Verification items for the finished model (mm, model axes). A direction names the side the tool comes from. Give positions to 0.01 mm unless a question says otherwise; leave off trailing zeros. Loops run counter-clockwise (first coordinate to the right, second up) from the corner with the lowest first, then second, coordinate; pieces in that order, holes last. Notation, with made-up numbers: M 24.5,-38.75 L 56.5,-38.75 A31 ccw 56.5,-9.75 Z; hole C 78,-37.5 d3. An arc over 180 degrees is marked long. Put each result on its own line as item: value. Start each with the question number.
from build123d import *

# Parameters (mm, degrees)
SKETCH1_R             = 60
BOSS_EXTRUDE1_DEPTH   = 19
SKETCH2_R             = 55
SKETCH2_R_2           = 50
CUT_EXTRUDE1_DEPTH    = 5
SKETCH6_W             = 17.5
SKETCH6_H             = 14
M6_TAPPED_HOLE1_D     = 5
M6_TAPPED_HOLE1_DEPTH = 15
M6_TAPPED_HOLE1_TIP   = 1.502151548


with BuildPart() as part:
    # Sketch1 → Boss-Extrude1 (new body)
    with BuildSketch(Plane(origin=(0, 0, 0), x_dir=(1, 0, 0), z_dir=(0, 1, 0))):
        with Locations(Location((0, 0, 0), (0, 0, 270))):
            Circle(SKETCH1_R)
    extrude(amount=BOSS_EXTRUDE1_DEPTH)

    # Sketch2 → Cut-Extrude1 (cut)
    with BuildSketch(Plane(origin=(0, 19, 0), x_dir=(1, 0, 0), z_dir=(0, 1, 0))):
        with Locations(Location((0, 0, 0), (0, 0, 270))):
            Circle(SKETCH2_R)
        with Locations(Location((0, 0, 0), (0, 0, 270))):
            Circle(SKETCH2_R_2, mode=Mode.SUBTRACT)
    extrude(amount=-CUT_EXTRUDE1_DEPTH, mode=Mode.SUBTRACT)

    # Sketch4 → Cut-Revolve1 (revolve, cut)
    with BuildSketch(Plane.XY, mode=Mode.PRIVATE) as cut_revolve1_sk:
        Polygon((45, 19), (45, 3.5), (40, 3.5), (40, 2.5), (0, 2.5), (0, 19), align=None)
    revolve(cut_revolve1_sk.sketch.rotate(Axis((0, 0, 0), (0, 1, 0)), 90), axis=Axis((0, 0, 0), (0, 1, 0)), mode=Mode.SUBTRACT)

    # Sketch5 → Revolve1 (revolve)
    with BuildSketch(Plane.XY, mode=Mode.PRIVATE) as revolve1_sk:
        Polygon((17.5, 0), (17.5, 14), (11, 14), (11, 19), (24, 19), (24, 0), align=None)
    revolve(revolve1_sk.sketch.rotate(Axis((0, 0, 0), (0, 1, 0)), 90), axis=Axis((0, 0, 0), (0, 1, 0)))

    # Sketch6 → Cut-Revolve2 (revolve, cut)
    with BuildSketch(Plane.XY, mode=Mode.PRIVATE) as cut_revolve2_sk:
        with Locations((8.75, 7)):
            Rectangle(SKETCH6_W, SKETCH6_H)
    revolve(cut_revolve2_sk.sketch.rotate(Axis((0, 0, 0), (0, 1, 0)), 90), axis=Axis((0, 0, 0), (0, 1, 0)), mode=Mode.SUBTRACT)

    # M6 Tapped Hole1
    with Locations(Plane(origin=(0, 19, 0), x_dir=(1, 0, 0), z_dir=(0, 1, 0))):
        with Locations((50.71110588, 13.587999868), (50.71110588, -13.587999868)):
            Hole(M6_TAPPED_HOLE1_D / 2, depth=M6_TAPPED_HOLE1_DEPTH)
            with Locations((0, 0, -(M6_TAPPED_HOLE1_DEPTH + M6_TAPPED_HOLE1_TIP / 2))):  # 118° drill point
                Cone(0, M6_TAPPED_HOLE1_D / 2, M6_TAPPED_HOLE1_TIP, mode=Mode.SUBTRACT)


solid = part.part
Q1. Go/stop test with flat-tipped pins: pin 1 (5 mm diameter, centred on x = -27.5, y = 6.5, fed in from +Z); pin 2 (5 mm diameter, centred on y = 17, z = 33, fed in from +X); pin 3 (8 mm diameter, centred on y = 17, z = -10, fed in from +X). Record where each tip stops, or that it passes through.
Q2. Scan lines: L1, parallel to X at y = 7, z = 0; L2, parallel to Z at x = -31.5, y = 18.25; L3, parallel to X at y = 7.5, z = -11. Record each from-to range of solid material in increasing order.
Q3. Release check for a two-part mould opening along Z. For faces 1 (the face through (5, 19, 10)), 2 (the face through (51.11, 2.76, -13.42)), 3 (the face through (15.02, 16.54, 47.69)), 4 (the face through (2.64, 9.37, -59.94)) record: pulls with the +Z half, pulls with the -Z half, needs draft (parallel to the pull), parting line crosses it, or undercut.
Q4. Cross-section at D-D, the plane x = -12.5. Record the boundary of the cut face in (y, z).
Q5. Cross-section at C-C, the plane y = 7.75. Record the boundary of the cut face in (x, z), then the cut area to 3 significant figures.
Q6. Set-up check for faces 5 (the face through (17.084, 7.098, 3.794)), 6 (the face through (-49, 19, 26)), 7 (the face through (-7.21, 10.63, -22.89)): record each of +Z, -Z, +X, -X, +Y, -Y from which the full face is reachable in a straight line by a thin tool's end or side.
Ans:
1. pin 1: stops at z = 54.54
1. pin 2: stops at x = 51.67
1. pin 3: stops at x = 59.7
2. L1: x = -60 to -45, -24 to -17.5, 17.5 to 24, 45 to 60
2. L2: z = -51.07 to -45.09, -38.83 to -32.14, 32.14 to 38.83, 45.09 to 51.07
2. L3: x = -58.98 to -43.63, -21.33 to -13.61, 13.61 to 21.33, 43.63 to 58.98
3. face 1: needs draft
3. face 2: undercut
3. face 3: undercut
3. face 4: parting line crosses it
4. outline: M 0,-58.68 L 19,-58.68 L 19,-53.56 L 14,-53.56 L 14,-48.41 L 19,-48.41 L 19,-43.23 L 3.5,-43.23 L 3.5,-38 L 2.5,-38 L 2.5,-20.49 L 19,-20.49 L 19,20.49 L 2.5,20.49 L 2.5,38 L 3.5,38 L 3.5,43.23 L 19,43.23 L 19,48.41 L 14,48.41 L 14,53.56 L 19,53.56 L 19,58.68 L 0,58.68 L 0,12.25 L 14,12.25 L 14,-12.25 L 0,-12.25 Z
5. outline: C 0,0 d120; C 0,0 d48; hole C 0,0 d90; hole C 0,0 d35; hole C 50.71,-13.59 d5; hole C 50.71,13.59 d5
5. area: 5,760 mm^2
6. face 5: -Y
6. face 6: +Z, -Z, +X, -X, +Y
6. face 7: +Y
